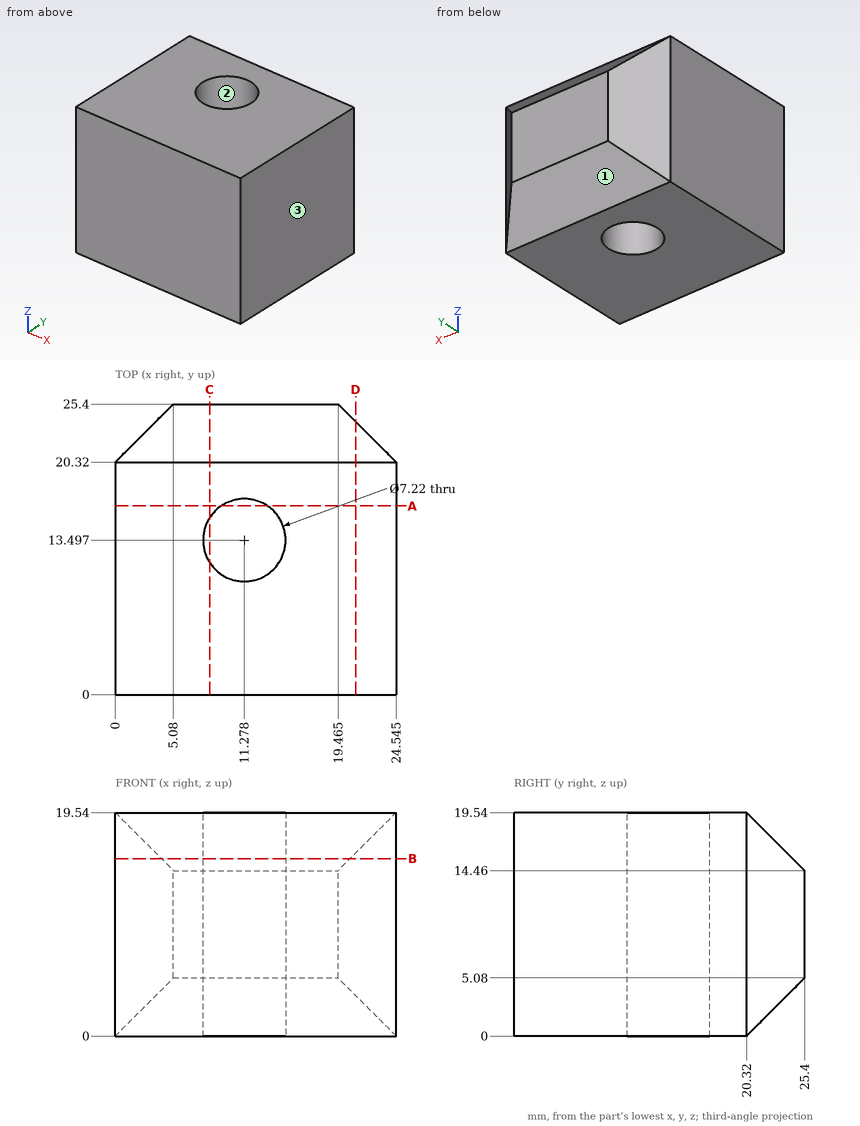
Design review of the part shown in the three views and the two pictorial views. Dimensions are in mm from the part's minimum x, y and z. Give positions to 0.01 mm unless a question says otherwise; leave off trailing zeros. Write each loop counter-clockwise with the first axis right and the second up, starting at its lowest first coordinate (ties: lowest second). Pieces come first, ordered by that corner, then holes. Notation, with made-up numbers: (59.25, -22) -> (108.25, -22) arc R28 ccw to (108.25, 3) -> close; hole circle Ø11 at (11.5, 59). An arc over 180 degrees is marked (long way). Answer in a Markdown table with one row per item.
1) Add section B-B on z = 15.5. State the section outline as (x, y) points (1 decimal), plus the area to 3 significant figures.
Worked answers:
| item | result |
|---|---|
| outline | (0, 0) -> (24.5, 0) -> (24.5, 20.3) -> (20.5, 24.4) -> (4, 24.4) -> (0, 20.3) -> close; hole circle Ø7.2 at (11.3, 13.5) |
| area | 541 mm² |
2) Clearance check with flat-ended pins moving along their axes: P1, Ø6, axis at x = 6, z = 7, coming from the -Y side; P2, Ø4.5, axis at x = 11.28, y = 13.5, coming from the +Z side. State where each tip first meets the part, or that it passes through.
Worked answers:
| item | result |
|---|---|
| P1 | y = 0 |
| P2 | through |
3) Add section A-A on y = 16.5. State the section outline as (x, z) points (1 decimal).
Worked answers:
| item | result |
|---|---|
| outline | (0, 0) -> (9.3, 0) -> (9.3, 19.5) -> (0, 19.5) -> close; (13.3, 0) -> (24.5, 0) -> (24.5, 19.5) -> (13.3, 19.5) -> close |
4) Mouldability with a two-part tool opening along X and no side actions: class the marked faces 1, 2 and 3 as +X half, -X half, draft (parallel to the pull), parting line (faces both ways), or undercut.
Worked answers:
| item | result |
|---|---|
| face 1 | draft |
| face 2 | undercut |
| face 3 | +X half |
5) Add section C-C on x = 8.25. State the section outline as (y, z) points, plus the area to 3 significant figures.
Worked answers:
| item | result |
|---|---|
| outline | (0, 0) -> (11.53, 0) -> (11.53, 19.54) -> (0, 19.54) -> close; (15.46, 0) -> (20.32, 0) -> (25.4, 5.08) -> (25.4, 14.46) -> (20.32, 19.54) -> (15.46, 19.54) -> close |
| area | 394 mm² |
6) Add section D-D on x = 21. State the section outline as (y, z) points (1 decimal).
Worked answers:
| item | result |
|---|---|
| outline | (0, 0) -> (20.3, 0) -> (23.9, 3.5) -> (23.9, 16) -> (20.3, 19.5) -> (0, 19.5) -> close |
7) For L1, parallel to Y at x = 14.5, z = 3.25 (1 decimal); L2, parallel to X at y = 14.25, z = 16 (1 decimal); L3, parallel to Y at x = 3, z = 10.5, list the stretches that pass through material, from the lowest coordinate up. Write a range as [from, to].
Worked answers:
| item | result |
|---|---|
| L1 | [0, 11.9], [15.1, 23.6] |
| L2 | [0, 7.7], [14.8, 24.5] |
| L3 | [0, 23.32] |
